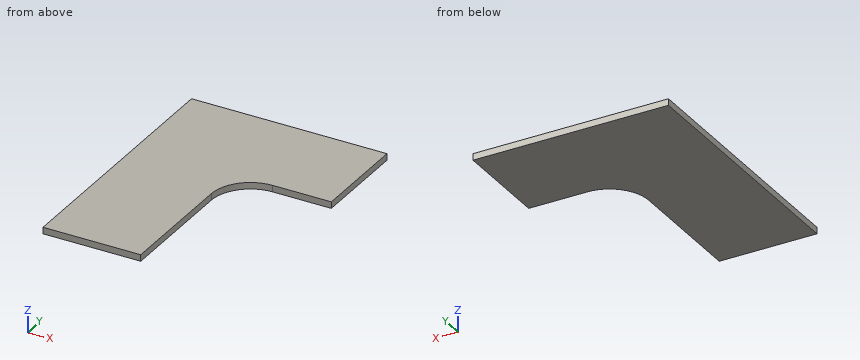
from build123d import *

# Parameters (mm, degrees)
F9_DEPTH = 50


# Not quite as in the source:
# - the program builds the solid bodies; features that only make, move or delete a surface that nothing else refers to are left out


with BuildPart() as f9:
    # F3 (on offset) → F9 (new body)
    with BuildSketch(Plane.XY.offset(750)):
        with BuildLine():
            ThreePointArc((0, -300), (87.867965644, -87.867965644), (300, 0))
            Line((300, 0), (750, 0))
            Line((750, 0), (750, 750))
            Line((750, 750), (-750, 750))
            Line((-750, 750), (-750, -1250))
            Line((-750, -1250), (0, -1250))
            Line((0, -1250), (0, -300))
        make_face()
    extrude(amount=-F9_DEPTH)


solid = f9.part
Verification items for the finished model (mm, model axes). Coordinates: 2 decimals unless noted, no trailing zeros. Order: outer loops, then holes, each group sorted by start corner. A loop starts at its lowest first (then second) coordinate and runs counter-clockwise, first axis right, second up. Notation, with made-up numbers: M 62,60 L 70,60 A24 ccw 70,96 Z; hole C 85.25,46 d10. An arc over 180 degrees is marked long. One line per item, written item: value. Start each with the question number.
Item 1: Scan lines: probe 1 along X at (y, z) = (-586.5, 718); probe 2 along Y at (x, z) = (594, 731); probe 3 along X at (y, z) = (-227.5, 707). Record each from-to range of solid material in increasing order.
Item 2: Sectioned sample at C-C (y = -662.5). Enter the section's corners in (x, z), then the cut area to 3 significant figures.
Item 3: Gauge pin test, flat end, axial feed: pin 1 (1 mm diameter, centred on x = 80.5, z = 741, fed in from -Y). Record the tip position at first contact, or that the pin passes through.
Item 4: Sectioned sample at B-B (x = 275). Enter the section's corners in (y, z).
Item 5: Sectioned sample at A-A (z = 738). Enter the section's corners in (x, y).
Conclusion:
1. probe 1: x = -750 to 0
1. probe 2: y = 0 to 750
1. probe 3: x = -750 to 8.89
2. outline: M -750,700 L 0,700 L 0,750 L -750,750 Z
2. area: 37,500 mm^2
3. pin 1: stops at y = -96.04
4. outline: M -1.04,700 L 750,700 L 750,750 L -1.04,750 Z
5. outline: M -750,-1250 L 0,-1250 L 0,-300 A300 cw 300,0 L 750,0 L 750,750 L -750,750 Z
